Could you check a few things on this model? Use its own coordinates, in mm. A direction names the side the tool comes from. Give positions to 0.01 mm unless a question says otherwise; leave off trailing zeros. Write each loop counter-clockwise with the first axis right and the second up, starting at its lowest first coordinate (ties: lowest second). Pieces come first, ordered by that corner, then holes. Notation, with made-up numbers: M -24,-38 L 20,-38 A36 cw 20,-1 Z; hole C 71,24 d1. An arc over 180 degrees is marked long. One line per item, written item: value.
```python
from build123d import *

# Parameters (mm, degrees)
SKETCH011_W     = 82
SKETCH011_H     = 78
SKETCH011_R     = 7.485
SKETCH011_R_2   = 5.3
PAD011_DEPTH    = 15
SKETCH012_W     = 7.5
SKETCH012_H     = 6
PAD012_DEPTH    = 6
SKETCH013_R     = 1.5
POCKET003_DEPTH = 3
SKETCH014_R     = 1.5
POCKET004_DEPTH = 3
SKETCH015_R     = 1.5
POCKET005_DEPTH = 6
SKETCH016_R     = 1.5
POCKET006_DEPTH = 6
SKETCH023_W     = 17.6
SKETCH023_H     = 23
POCKET012_DEPTH = 15.001


with BuildPart() as part:
    # Sketch011 → Pad011 (new body)
    with BuildSketch(Plane.XZ):
        with Locations((0, 39)):
            Rectangle(SKETCH011_W, SKETCH011_H)
        with Locations((26.05, 29.15)):
            Circle(SKETCH011_R, mode=Mode.SUBTRACT)
        with Locations((-8.85, 29.15)):
            Circle(SKETCH011_R_2, mode=Mode.SUBTRACT)
    extrude(amount=PAD011_DEPTH)

    # Sketch012 (on Face8 of Pad011) → Pad012 (join)
    with BuildSketch(Plane.XZ.offset(15)):
        with Locations((-19.65, 3)):
            Rectangle(SKETCH012_W, SKETCH012_H)
        with Locations((-19.65, 75)):
            Rectangle(SKETCH012_W, SKETCH012_H)
        with Locations((13.065, 10)):
            Rectangle(SKETCH012_W, SKETCH012_H)
        with Locations((13.065, 69)):
            Rectangle(SKETCH012_W, SKETCH012_H)
    extrude(amount=PAD012_DEPTH)

    # Sketch013 (on Face11 of Pad012) → Pocket003 (cut)
    with BuildSketch(Plane(origin=(0, 0, 6), x_dir=(-1, 0, 0), z_dir=(0, 0, 1))):
        with Locations((19.65, 18)):
            Circle(SKETCH013_R)
    extrude(amount=-POCKET003_DEPTH, mode=Mode.SUBTRACT)

    # Sketch014 (on Face16 of Pocket003) → Pocket004 (cut)
    with BuildSketch(Plane(origin=(0, 0, 13), x_dir=(-1, 0, 0), z_dir=(0, 0, 1))):
        with Locations((-13.065, 18)):
            Circle(SKETCH014_R)
    extrude(amount=-POCKET004_DEPTH, mode=Mode.SUBTRACT)

    # Sketch015 (on Face6 of Pocket004) → Pocket005 (cut)
    with BuildSketch(Plane(origin=(0, 0, 78), x_dir=(-1, 0, 0), z_dir=(0, 0, 1))):
        with Locations((19.65, 18)):
            Circle(SKETCH015_R)
    extrude(amount=-POCKET005_DEPTH, mode=Mode.SUBTRACT)

    # Sketch016 (on Face20 of Pocket005) → Pocket006 (cut)
    with BuildSketch(Plane(origin=(0, 0, 72), x_dir=(-1, 0, 0), z_dir=(0, 0, 1))):
        with Locations((-13.065, 18)):
            Circle(SKETCH016_R)
    extrude(amount=-POCKET006_DEPTH, mode=Mode.SUBTRACT)

    # Sketch023 (on Face5 of Pocket006) → Pocket012 (cut, through all)
    with BuildSketch(Plane.XZ.offset(15)):
        with Locations((-32.2, 66.5)):
            Rectangle(SKETCH023_W, SKETCH023_H)
    extrude(amount=-POCKET012_DEPTH, mode=Mode.SUBTRACT)


with BuildPart() as part_1:
    # Body002 placement: moved
    add(part.part.moved(Location((0, -39, 0))))


solid = part_1.part
```
1) If we section it at A-A, the plane x = -19.65: Write out the boundary of the cut face in (y, z), then the cut area to 4 significant figures.
Outcome:
outline: M -60,0 L -39,0 L -39,78 L -55.5,78 L -55.5,72 L -54,72 L -54,6 L -55.5,6 L -55.5,3 L -58.5,3 L -58.5,6 L -60,6 Z; M -60,72 L -58.5,72 L -58.5,78 L -60,78 Z
area: 1,215 mm^2
2) On a 3-axis mill with a long thin cutter (end or side, diameter ignored), from which of +Z, -Z, +X, -X, +Y, -Y can I reach the whole of each face in a straight line? I mean faces 1 (the face through (-20.456, -58.265, 75.042)), 2 (the face through (9.315, -57, 69)), 3 (the face through (15, -57, 13)). Say none if no direction works.
Outcome:
face 1: +Z
face 2: +Z, -Z, -X, -Y
face 3: +X, -X, -Y
3) If we section it at D-D, the plane y = -40.25: Write out the boundary of the cut face in (x, z) (3 decimals).
Outcome:
outline: M -41,0 L 41,0 L 41,78 L -23.4,78 L -23.4,55 L -41,55 Z; hole C -8.85,29.15 d10.6; hole C 26.05,29.15 d14.97
4) If we section it at C-C, the plane y = -57: Give the number of separate pieces and of enclosed holes in the cut face, then the cut area to 3 significant figures.
Outcome:
separate pieces: 6
enclosed holes: 0
area: 126 mm^2
5) Please list where these lines run through material, in increasing order: L1, parallel to Z at x = 26.05, y = -42.5 (3 decimals); L2, parallel to X at y = -57, z = 75.8; L3, parallel to Z at x = 10.5, y = -55.5. Write a range as from..to.
Outcome:
L1: z = 0..21.665, 36.635..78
L2: x = -23.4..-21.15, -18.15..-15.9
L3: z = 7..13, 66..72
6) If we section it at B-B, the plane z = 29.15: Write out the boundary of the cut face in (x, y) (3 decimals), then the cut area to 3 significant figures.
Outcome:
outline: M -41,-54 L -14.15,-54 L -14.15,-39 L -41,-39 Z; M -3.55,-54 L 18.565,-54 L 18.565,-39 L -3.55,-39 Z; M 33.535,-54 L 41,-54 L 41,-39 L 33.535,-39 Z
area: 846 mm^2
7) We'd pull the mould along Y, two halves only. Please class faces 4 (the face through (-3.954, -46.395, 27.12)), 5 (the face through (-1, -39, 40)), 6 (the face through (12.259, -58.265, 69.042)), 7 (the face through (13, -57, 10)): pulls with the +Y half, pulls with the -Y half, needs draft (parallel to the pull), parting line crosses it, or undercut.
Outcome:
face 4: needs draft
face 5: pulls with the +Y half
face 6: undercut
face 7: undercut
8) I'm going to push flat-ended pins straight in: pin 1 (10.5 mm diameter, centred on y = -49.5, z = 63.5, fed in from -X); pin 2 (1.8 mm diameter, centred on x = 14, y = -57, fed in from +Z); pin 3 (2.5 mm diameter, centred on x = 13.065, y = -57, fed in from -Z); pin 4 (6.5 mm diameter, centred on x = -8.85, z = 29.15, fed in from +Y). Where does each tip first touch, or does it pass through?
Outcome:
pin 1: stops at x = -23.4
pin 2: stops at z = 72
pin 3: stops at z = 7
pin 4: passes through
